from build123d import *

# Parameters (mm, degrees)
SKETCH1_R           = 38.1
BOSS_EXTRUDE1_DEPTH = 152.4


with BuildPart() as part:
    # Sketch1 → Boss-Extrude1 (new body)
    with BuildSketch(Plane.XY):
        Polygon((304.8, -304.8), (304.8, 304.8), (127, 304.8), (127, 50.8), (-127, 50.8), (-127, 304.8), (-304.8, 304.8), (-304.8, -304.8), align=None)
        with Locations(Location((-224.8, 224.8, 0), (0, 0, 180))):
            Circle(SKETCH1_R, mode=Mode.SUBTRACT)
        with Locations(Location((224.8, 224.8, 0), (0, 0, 180))):
            Circle(SKETCH1_R, mode=Mode.SUBTRACT)
    extrude(amount=BOSS_EXTRUDE1_DEPTH)


solid = part.part
Here's how the part is built. I have some questions about the finished solid (model axes, mm). A direction names the side the tool comes from. Round coordinates to 2 decimals unless told otherwise and drop trailing zeros. Write each loop counter-clockwise with the first axis right and the second up, starting at its lowest first coordinate (ties: lowest second). Pieces come first, ordered by that corner, then holes.
1. Suppose I cut it at D-D (y = 224.8). List the corners of the cut face in (x, z) for me, and give its area (3 significant figures).
2. Suppose I cut it at C-C (z = 44.5). List the corners of the cut face in (x, y) for me.
3. I need wall thicknesses on L1, parallel to X at y = 224.8, z = 121.5; L2, parallel to X at y = 242.5, z = 83; L3, parallel to X at y = 57, z = 112.5. Which ranges of each line are inside material? Lowest first, please.
4. If we mould it in two halves opening along X, with no side actions, what happens to faces 3 (the flat face through (-304.8, 4, 75)), 4 (the flat face through (-215, 304.8, 75)), 5 (the cylindrical face through (262.863, 223.125, 75.133))? For each: released by +X, released by -X, zero draft, split by the parting line, or undercut.
5. Suppose I cut it at B-B (x = 224.8). List the corners of the cut face in (y, z) for me.
6. For faces 1 (the flat face through (2, 50.8, 75)), 2 (the flat face through (217, 304.8, 75)), which set-ups out of +Z, -Z, +X, -X, +Y, -Y let a thin tool reach every point of the face, with its end or its side?
7. Suppose I cut it at A-A (y = 152). List the corners of the cut face in (x, z) for me, and give its area (3 significant figures).
Answer sheet:
1. outline: (-304.8, 0) - (-262.9, 0) - (-262.9, 152.4) - (-304.8, 152.4) - close; (-186.7, 0) - (-127, 0) - (-127, 152.4) - (-186.7, 152.4) - close; (127, 0) - (186.7, 0) - (186.7, 152.4) - (127, 152.4) - close; (262.9, 0) - (304.8, 0) - (304.8, 152.4) - (262.9, 152.4) - close
1. area: 31,000 mm2
2. outline: (-304.8, -304.8) - (304.8, -304.8) - (304.8, 304.8) - (127, 304.8) - (127, 50.8) - (-127, 50.8) - (-127, 304.8) - (-304.8, 304.8) - close; hole circle Ø76.2 at (-224.8, 224.8); hole circle Ø76.2 at (224.8, 224.8)
3. L1: x = -304.8 to -262.9, -186.7 to -127, 127 to 186.7, 262.9 to 304.8
3. L2: x = -304.8 to -258.54, -191.06 to -127, 127 to 191.06, 258.54 to 304.8
3. L3: x = -304.8 to -127, 127 to 304.8
4. face 3: released by -X
4. face 4: zero draft
4. face 5: undercut
5. outline: (-304.8, 0) - (186.7, 0) - (186.7, 152.4) - (-304.8, 152.4) - close; (262.9, 0) - (304.8, 0) - (304.8, 152.4) - (262.9, 152.4) - close
6. face 1: +Z, -Z, +Y
6. face 2: +Z, -Z, +X, -X, +Y
7. outline: (-304.8, 0) - (-127, 0) - (-127, 152.4) - (-304.8, 152.4) - close; (127, 0) - (304.8, 0) - (304.8, 152.4) - (127, 152.4) - close
7. area: 54,200 mm2
